from build123d import *

# Parameters (mm, degrees)
CROQUIS1_W              = 128
CROQUIS1_H              = 98
CROQUIS1_W_2            = 118
CROQUIS1_H_2            = 88
SALIENTE_EXTRUIR5_DEPTH = 30
CROQUIS6_W              = 128
CROQUIS6_H              = 98
SALIENTE_EXTRUIR6_DEPTH = 5
CROQUIS7_W              = 40
CROQUIS7_H              = 20
CORTAR_EXTRUIR2_DEPTH   = 10
REDONDEO1_R             = 10
CROQUIS8_R              = 2
CORTAR_EXTRUIR3_DEPTH   = 10
SALIENTE_EXTRUIR7_DEPTH = 13
CROQUIS11_R             = 5
CORTAR_EXTRUIR4_DEPTH   = 60
CROQUIS12_R             = 7.5
CROQUIS12_R_2           = 5
SALIENTE_EXTRUIR9_DEPTH = 10


with BuildPart() as part:
    # Croquis1 → Saliente-Extruir5 (new body)
    with BuildSketch(Plane(origin=(0, 0, 0), x_dir=(1, 0, 0), z_dir=(0, 1, 0))):
        Rectangle(CROQUIS1_W, CROQUIS1_H)
        Rectangle(CROQUIS1_W_2, CROQUIS1_H_2, mode=Mode.SUBTRACT)
    extrude(amount=SALIENTE_EXTRUIR5_DEPTH)

    # Croquis6 → Saliente-Extruir6 (add)
    with BuildSketch(Plane(origin=(0, 30, 0), x_dir=(1, 0, 0), z_dir=(0, 1, 0))):
        Rectangle(CROQUIS6_W, CROQUIS6_H)
    extrude(amount=-SALIENTE_EXTRUIR6_DEPTH)

    # Croquis7 → Cortar-Extruir2 (cut)
    with BuildSketch(Plane(origin=(0, 30, 0), x_dir=(1, 0, 0), z_dir=(0, 1, 0))):
        with Locations((26.740101048, 0)):
            Rectangle(CROQUIS7_W, CROQUIS7_H)
    extrude(amount=-CORTAR_EXTRUIR2_DEPTH, mode=Mode.SUBTRACT)

    # Redondeo1
    redondeo1_edges = [part.edges().sort_by_distance(p)[0] for p in [
        (-64, 15, 49),
        (-64, 15, -49),
    ]]
    fillet(redondeo1_edges, radius=REDONDEO1_R)

    # Croquis8 → Cortar-Extruir3 (cut)
    with BuildSketch(Plane(origin=(0, 30, 0), x_dir=(1, 0, 0), z_dir=(0, 1, 0))):
        with Locations((50.740101048, -5)):
            Circle(CROQUIS8_R)
        with Locations((50.740101048, 5)):
            Circle(CROQUIS8_R)
        with Locations((2.740101048, 5)):
            Circle(CROQUIS8_R)
        with Locations((2.740101048, -5)):
            Circle(CROQUIS8_R)
    extrude(amount=-CORTAR_EXTRUIR3_DEPTH, mode=Mode.SUBTRACT)

    # Croquis9 → Saliente-Extruir7 (add)
    with BuildSketch(Plane(origin=(0, 30, 0), x_dir=(1, 0, 0), z_dir=(0, 1, 0))):
        with BuildLine():
            Line((16.584456677, 10), (19.419592972, 10))
            ThreePointArc((19.419592972, 10), (56.740101048, 0), (19.419592972, -10))
            Line((19.419592972, -10), (16.584456677, -10))
            ThreePointArc((16.584456677, -10), (59.240101048, 0), (16.584456677, 10))
        make_face()
    extrude(amount=SALIENTE_EXTRUIR7_DEPTH)

    # Croquis11 → Cortar-Extruir4 (cut)
    with BuildSketch(Plane(origin=(0, 30, 0), x_dir=(1, 0, 0), z_dir=(0, 1, 0))):
        with Locations((-49.972168211, 0)):
            Circle(CROQUIS11_R)
    extrude(amount=-CORTAR_EXTRUIR4_DEPTH, mode=Mode.SUBTRACT)

    # Croquis12 → Saliente-Extruir9 (add)
    with BuildSketch(Plane(origin=(0, 30, 0), x_dir=(1, 0, 0), z_dir=(0, 1, 0))):
        with Locations((-49.972168211, 0)):
            Circle(CROQUIS12_R)
        with Locations((-49.972168211, 0)):
            Circle(CROQUIS12_R_2, mode=Mode.SUBTRACT)
    extrude(amount=SALIENTE_EXTRUIR9_DEPTH)


solid = part.part
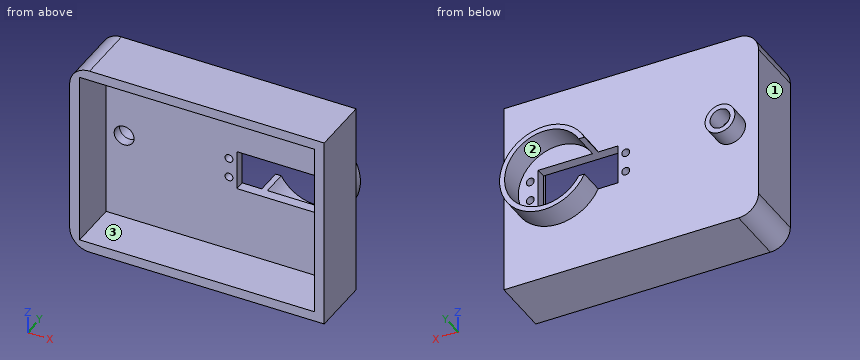
The model under review builds one solid part; all positions refer to its coordinate system, in mm. Face numbers are marked on the shaded views. A direction names the side the tool comes from. Round coordinates to 2 decimals unless told otherwise and drop trailing zeros. Order: outer loops, then holes, each group sorted by start corner. A loop starts at its lowest first (then second) coordinate and runs counter-clockwise, first axis right, second up. Notation, with made-up numbers: (51.25, 35) -> (58.25, 35) arc R14 ccw to (58.25, 45) -> close; hole circle Ø1 at (8, 14). An arc over 180 degrees is marked (long way). Return JSON: item names as keys, results as strings.
1. Take a section at A-A (z = 0). Write out the cut boundary in (x, y).
Answer block:
{"outline": "(-64, 0) -> (-59, 0) -> (-59, 25) -> (-54.97, 25) -> (-54.97, 40) -> (-57.47, 40) -> (-57.47, 30) -> (-64, 30) -> close; (-44.97, 25) -> (6.74, 25) -> (6.74, 30) -> (-42.47, 30) -> (-42.47, 40) -> (-44.97, 40) -> close; (46.74, 25) -> (59, 25) -> (59, 0) -> (64, 0) -> (64, 30) -> (59.24, 30) -> (59.24, 43) -> (56.74, 43) -> (56.74, 30) -> (46.74, 30) -> close"}
2. For the marked faces 1, 2 and 3, list the 3-axis set-ups (+Z, -Z, +X, -X, +Y, -Y) from which the entire face can be reached by the end or side of a thin tool; tool diameter is ignored.
Answer block:
{"face 1": "+Z, -Z, -X, +Y, -Y", "face 2": "+Y", "face 3": "-Y"}
3. Take a section at D-D (x = 23.5). Write out the cut boundary in (y, z).
Answer block:
{"outline": "(0, -49) -> (30, -49) -> (30, -18.19) -> (43, -18.19) -> (43, -14.99) -> (30, -14.99) -> (30, -10) -> (25, -10) -> (25, -44) -> (0, -44) -> close; (0, 44) -> (25, 44) -> (25, 10) -> (30, 10) -> (30, 14.99) -> (43, 14.99) -> (43, 18.19) -> (30, 18.19) -> (30, 49) -> (0, 49) -> close"}
4. Take a section at C-C (y = 20). Write out the cut boundary in (x, z).
Answer block:
{"outline": "(-64, -39) arc R10 ccw to (-54, -49) -> (64, -49) -> (64, 49) -> (-54, 49) arc R10 ccw to (-64, 39) -> close; hole (-59, -44) -> (59, -44) -> (59, 44) -> (-59, 44) -> close"}
5. Take a section at B-B (y = 35). Write out the cut boundary in (x, z).
Answer block:
{"outline": "circle Ø15 at (-49.97, 0); (16.58, -10) arc R22.5 ccw (long way) to (16.58, 10) -> (19.42, 10) arc R20 cw (long way) to (19.42, -10) -> close; hole circle Ø10 at (-49.97, 0)"}
6. For L1, parallel to X at y = 27.3, z = 0; L2, parallel to Z at x = 53, y = 23; L3, parallel to X at y = 37, z = 0, list the stretches that pass through material, from the lowest coordinate up. Write a range as [from, to].
Answer block:
{"L1": "x = [-64, -54.97], [-44.97, 6.74], [46.74, 64]", "L2": "z = [-49, -44], [44, 49]", "L3": "x = [-57.47, -54.97], [-44.97, -42.47], [56.74, 59.24]"}
7. Insertion check: P1, Ø3.5, axis at x = 2.74, z = -5, coming from the -Y side; P2, Ø16.5, axis at x = -52.5, z = 3.5, coming from the +Y side; P3, Ø5, axis at x = -26, z = -5, coming from the -Y side; P4, Ø8, axis at x = 27.5, z = -25, coming from the +Y side. Each pin has a flat end and moves straight along its axis. Give the tip position at first contact, or say it passes through.
Answer block:
{"P1": "passes through", "P2": "stops at y = 40", "P3": "stops at y = 25", "P4": "stops at y = 30"}
